Source: CAD feature listing. Evaluate the final solid. Frame: model axes, mm. Round coordinates to 2 decimals unless told otherwise and drop trailing zeros. Write each loop counter-clockwise with the first axis right and the second up, starting at its lowest first coordinate (ties: lowest second). Pieces come first, ordered by that corner, then holes. Notation, with made-up numbers: M 68,9 L 120,9 A22 ccw 120,24 Z; hole C -19.5,-4 d1. An arc over 180 degrees is marked long. Use a Markdown table: item, result.
```python
from build123d import *

# Parameters (mm, degrees)
BOX006_W     = 650
BOX006_H     = 30
BOX006_DEPTH = 30
BOX007_W     = 650
BOX007_H     = 30
BOX007_DEPTH = 30
BOX008_W     = 30
BOX008_H     = 650
BOX008_DEPTH = 30
BOX005_W     = 30
BOX005_H     = 650
BOX005_DEPTH = 30
BOX004_W     = 30
BOX004_H     = 30
BOX004_DEPTH = 525
BOX003_W     = 30
BOX003_H     = 30
BOX003_DEPTH = 525
BOX002_W     = 30
BOX002_H     = 30
BOX002_DEPTH = 525
BOX001_W     = 30
BOX001_H     = 30
BOX001_DEPTH = 525
BOX010_W     = 650
BOX010_H     = 30
BOX010_DEPTH = 30
BOX011_W     = 650
BOX011_H     = 30
BOX011_DEPTH = 30
BOX012_W     = 30
BOX012_H     = 650
BOX012_DEPTH = 30
BOX009_W     = 30
BOX009_H     = 650
BOX009_DEPTH = 30


with BuildPart() as box006:
    # Box006 → Box006 (new body)
    with BuildSketch(Plane.XY):
        with Locations((325, 15)):
            Rectangle(BOX006_W, BOX006_H)
    extrude(amount=BOX006_DEPTH)


with BuildPart() as box007:
    # Box007 → Box007 (new body)
    with BuildSketch(Plane(origin=(0, 620, 0), x_dir=(1, 0, 0), z_dir=(0, 0, 1))):
        with Locations((325, 15)):
            Rectangle(BOX007_W, BOX007_H)
    extrude(amount=BOX007_DEPTH)


with BuildPart() as box008:
    # Box008 → Box008 (new body)
    with BuildSketch(Plane(origin=(620, 0, 0), x_dir=(1, 0, 0), z_dir=(0, 0, 1))):
        with Locations((15, 325)):
            Rectangle(BOX008_W, BOX008_H)
    extrude(amount=BOX008_DEPTH)


with BuildPart() as obj1:
    # Box005 → Box005 (new body)
    with BuildSketch(Plane.XY):
        with Locations((15, 325)):
            Rectangle(BOX005_W, BOX005_H)
    extrude(amount=BOX005_DEPTH)

    # Fusion: union Box006, Box007, Box008
    add(box006.part)
    add(box007.part)
    add(box008.part)


with BuildPart() as box004:
    # Box004 → Box004 (new body)
    with BuildSketch(Plane(origin=(0, 620, 0), x_dir=(1, 0, 0), z_dir=(0, 0, 1))):
        with Locations((15, 15)):
            Rectangle(BOX004_W, BOX004_H)
    extrude(amount=BOX004_DEPTH)


with BuildPart() as box003:
    # Box003 → Box003 (new body)
    with BuildSketch(Plane(origin=(620, 620, 0), x_dir=(1, 0, 0), z_dir=(0, 0, 1))):
        with Locations((15, 15)):
            Rectangle(BOX003_W, BOX003_H)
    extrude(amount=BOX003_DEPTH)


with BuildPart() as box002:
    # Box002 → Box002 (new body)
    with BuildSketch(Plane(origin=(620, 0, 0), x_dir=(1, 0, 0), z_dir=(0, 0, 1))):
        with Locations((15, 15)):
            Rectangle(BOX002_W, BOX002_H)
    extrude(amount=BOX002_DEPTH)


with BuildPart() as box001:
    # Box001 → Box001 (new body)
    with BuildSketch(Plane.XY):
        with Locations((15, 15)):
            Rectangle(BOX001_W, BOX001_H)
    extrude(amount=BOX001_DEPTH)


with BuildPart() as box010:
    # Box010 → Box010 (new body)
    with BuildSketch(Plane.XY):
        with Locations((325, 15)):
            Rectangle(BOX010_W, BOX010_H)
    extrude(amount=BOX010_DEPTH)


with BuildPart() as box011:
    # Box011 → Box011 (new body)
    with BuildSketch(Plane(origin=(0, 620, 0), x_dir=(1, 0, 0), z_dir=(0, 0, 1))):
        with Locations((325, 15)):
            Rectangle(BOX011_W, BOX011_H)
    extrude(amount=BOX011_DEPTH)


with BuildPart() as box012:
    # Box012 → Box012 (new body)
    with BuildSketch(Plane(origin=(620, 0, 0), x_dir=(1, 0, 0), z_dir=(0, 0, 1))):
        with Locations((15, 325)):
            Rectangle(BOX012_W, BOX012_H)
    extrude(amount=BOX012_DEPTH)


with BuildPart() as parte_superior:
    # Box009 → Box009 (new body)
    with BuildSketch(Plane.XY):
        with Locations((15, 325)):
            Rectangle(BOX009_W, BOX009_H)
    extrude(amount=BOX009_DEPTH)

    # Fusion001: union Box010, Box011, Box012
    add(box010.part)
    add(box011.part)
    add(box012.part)


with BuildPart() as parte_superior_1:
    # Fusion001 placement: moved
    add(parte_superior.part.moved(Location((0, 0, 495))))

    # Fusion002: union obj1, Box004, Box003, Box002, Box001
    add(obj1.part)
    add(box004.part)
    add(box003.part)
    add(box002.part)
    add(box001.part)


solid = parte_superior_1.part
```
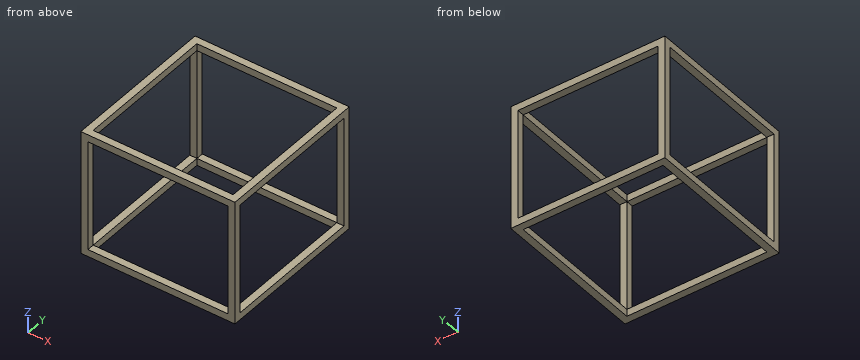
Q1. Section A-A on y = 366. Return loops of the section in (x, z), plus the area to 3 significant figures.
Results are:
| item | result |
|---|---|
| outline | M 0,0 L 30,0 L 30,30 L 0,30 Z; M 0,495 L 30,495 L 30,525 L 0,525 Z; M 620,0 L 650,0 L 650,30 L 620,30 Z; M 620,495 L 650,495 L 650,525 L 620,525 Z |
| area | 3,600 mm^2 |
Q2. Line query: L1, parallel to X at y = 456.5, z = 496. Output: solid intervals per line, ascending.
Results are:
| item | result |
|---|---|
| L1 | 0 to 30, 620 to 650 |
Q3. First-contact query: pin 1 Ø15 at (y, z) = (453, 515) entering from -X. Flat tip, straight axial feed; report the tip coordinate or a pass-through.
Results are:
| item | result |
|---|---|
| pin 1 | x = 0 |
